Read the model definition and answer for the solid it produces. Units are mm, in the model's axes. A direction names the side the tool comes from. Round coordinates to 2 decimals unless told otherwise and drop trailing zeros. Loops run counter-clockwise (first coordinate to the right, second up) from the corner with the lowest first, then second, coordinate; pieces in that order, holes last. Notation, with made-up numbers: M 73,84.25 L 130,84.25 A13 cw 130,107.25 Z; hole C 89,66.5 d9. An arc over 180 degrees is marked long. Answer as CSV lines item,"result".
Autodesk Inventor part; units mm, degrees
ref_plane "YZ Plane" through (0, 0, 0) normal (1, 0, 0) x (0, 1, 0)
ref_plane "XZ Plane" through (0, 0, 0) normal (0, 1, 0) x (-1, 0, 0)
ref_plane "XY Plane" through (0, 0, 0) normal (0, 0, 1) x (1, 0, 0)
sketch "Sketch1" plane through (0, 0, 0) normal (0, 0, 1) x (1, 0, 0)
  circle A0 centre (0, 0) radius 42.5
  line L0 (0, -42.5) -> (1000, -42.5)
  line L1 (1000, -42.5) -> (1000, -22.5)
  line L2 (1000, -22.5) -> (0, -22.5)
  line L3 (0, -22.5) -> (0, -42.5)
  line L4 (0, 42.5) -> (68, 42.5)
  line L5 (68, 42.5) -> (68, 22.5)
  line L6 (68, 22.5) -> (0, 22.5)
  line L7 (0, 22.5) -> (0, 42.5)
  circle A1 centre (0, 0) radius 22.5
  point P0 (0, -22.5)
  point P1 (0, 22.5)
  dimension "d0" = 85
  dimension "d1" = 20
  dimension "d2" = 20
  dimension "d4" = 1000
  dimension "d7" = 68
extrude "Extrusion1" add sketch "Sketch1" along normal blind 49 contours L7 A1 L3 A0 | L4 L5 L6 A0 | A0 L6 L7 | L3 L2 A0 | A0 L2 L1 L0
properties part number "J15BF.1.40_Yaxis"
1) Find section A-A, the plane z = 13.5. Give the vertices of the cut face in (x, y).
Evaluation:
outline,"M 0,-42.5 L 1000,-42.5 L 1000,-22.5 L 0,-22.5 A22.5 cw 0,22.5 L 68,22.5 L 68,42.5 L 0,42.5 A42.5 ccw Z"
2) A tool of negligible diameter and unlimited length cuts with its end or side. For faces 1 (the cylindrical face through (-42.49, -0.93, 24.16)), 2 (the flat face through (34, 22.5, 24)), 3 (the flat face through (68, 33, 24)), from which of +Z, -Z, +X, -X, +Y, -Y can it reach the whole face along a straight path? Write none if from no direction.
Evaluation:
face 1,"+Z, -Z, -X"
face 2,"+Z, -Z, +X"
face 3,"+Z, -Z, +X, +Y"
3) Each of these flat-tipped pins is pushed along its axis until it touches: P1, Ø4, axis at x = 94, z = 40, coming from the +Y side; P2, Ø12, axis at y = 1, z = 25, coming from the -X side; P3, Ø12, axis at y = -17.5, z = 9.5, coming from the -X side. Where does it stop, or does it pass through?
Evaluation:
P1,"stops at y = -22.5"
P2,"stops at x = -42.5"
P3,"stops at x = -40.91"
4) Straight lines are drawn through the part: line 1 (Y direction, x = 58, z = 25); line 2 (Y direction, x = 156.5, z = 22); line 3 (X direction, y = -3, z = 13.5). For each, find the intervals that lie inside material, in ascending order.
Evaluation:
line 1,"y = -42.5 to -22.5, 22.5 to 42.5"
line 2,"y = -42.5 to -22.5"
line 3,"x = -42.39 to -22.3"
5) Find section B-B, the plane y = 0. Give the vertices of the cut face in (x, z), then the cut area to 3 significant figures.
Evaluation:
outline,"M -42.5,0 L -22.5,0 L -22.5,49 L -42.5,49 Z"
area,"980 mm^2"
6) Determine the mould class of faces 4 (the flat face through (493, -42.5, 24)), 5 (the flat face through (1000, -33, 24)), 6 (the cylindrical face through (-22.495, -0.495, 24.157)) for opening direction Y: released by +Y, released by -Y, zero draft, split by the parting line, or undercut.
Evaluation:
face 4,"released by -Y"
face 5,"zero draft"
face 6,"undercut"
